Job drawing, mm, ordinate dimensions from the low corner. One solid piece. A direction names the side the tool comes from. Give positions to 0.01 mm unless a question says otherwise; leave off trailing zeros. Order: outer loops, then holes, each group sorted by start corner. A loop starts at its lowest first (then second) coordinate and runs counter-clockwise, first axis right, second up. Notation, with made-up numbers: (76, 37) -> (111, 37) arc R15 cw to (111, 44) -> close; hole circle Ø7 at (-4.75, 68). An arc over 180 degrees is marked (long way). Write item = value, one per line. Start each with the question number.
(1) Two-plate mould, pull along Y, no slides. Class the marked faces 3, 4 and 5: pulls with the +Y half, pulls with the -Y half, needs draft (parallel to the pull), parting line crosses it, or undercut.
(2) Saw through at B-B, the plane z = 4.2. List the corners of the cut face in (x, y), then the cut area to 3 significant figures.
(3) Probe line 1 along Y through (x, z) = (20, 0.2); line 2 along Y through (x, z) = (20, 1.6); line 3 along X through (y, z) = (29, 1.75) (1 decimal). List the from-to ranges inside material, lowest first. Write a range as from..to.
(4) Saw through at D-D, the plane x = 24. List the corners of the cut face in (y, z).
(5) Flat gauge pin, fed straight in: pin 1 (2 mm diameter, centred on y = 16.5, z = 4.5, fed in from -X). Where does the tip first touch, or does it go through?
(6) Saw through at A-A, the plane y = 20. List the corners of the cut face in (x, z).
(7) Saw through at C-C, the plane x = 20. List the corners of the cut face in (y, z).
(8) Which spindle directions (+Z, -Z, +X, -X, +Y, -Y) get a long thin tool onto all of the face, cutting with end or side? Do the marked faces 1 and 2. Say none if no direction does.
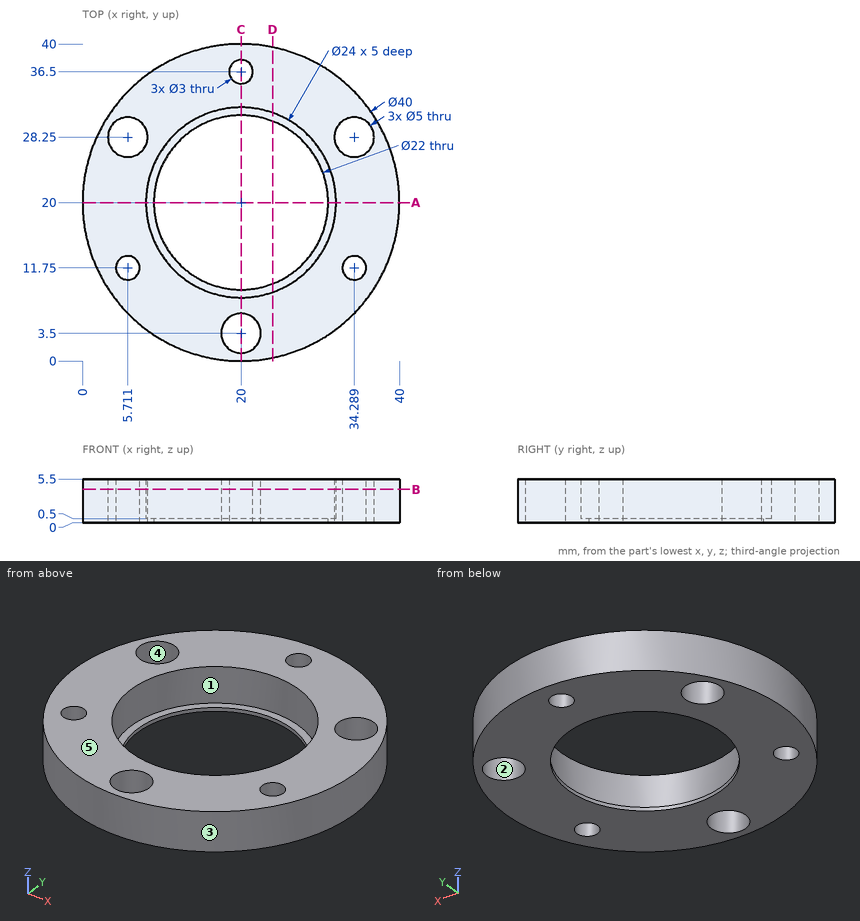
Results list:
q1.face_3 = parting line crosses it
q1.face_4 = undercut
q1.face_5 = needs draft
q2.outline = circle Ø40 at (20, 20); hole circle Ø5 at (5.71, 28.25); hole circle Ø3 at (5.71, 11.75); hole circle Ø24 at (20, 20); hole circle Ø5 at (20, 3.5); hole circle Ø3 at (20, 36.5); hole circle Ø5 at (34.29, 28.25); hole circle Ø3 at (34.29, 11.75)
q2.area = 724 mm^2
q3.line_1 = 0..1, 6..9, 31..35, 38..40
q3.line_2 = 0..1, 6..8, 32..35, 38..40
q3.line_3 = 2.1..3.3, 8.1..12.1, 27.9..31.9, 36.7..37.9
q4.outline = (0.4, 0) -> (9.75, 0) -> (9.75, 0.5) -> (8.69, 0.5) -> (8.69, 5.5) -> (0.4, 5.5) -> close; (30.25, 0) -> (39.6, 0) -> (39.6, 5.5) -> (31.31, 5.5) -> (31.31, 0.5) -> (30.25, 0.5) -> close
q5.pin_1 = 0.16
q6.outline = (0, 0) -> (9, 0) -> (9, 0.5) -> (8, 0.5) -> (8, 5.5) -> (0, 5.5) -> close; (31, 0) -> (40, 0) -> (40, 5.5) -> (32, 5.5) -> (32, 0.5) -> (31, 0.5) -> close
q7.outline = (0, 0) -> (1, 0) -> (1, 5.5) -> (0, 5.5) -> close; (6, 0) -> (9, 0) -> (9, 0.5) -> (8, 0.5) -> (8, 5.5) -> (6, 5.5) -> close; (31, 0) -> (35, 0) -> (35, 5.5) -> (32, 5.5) -> (32, 0.5) -> (31, 0.5) -> close; (38, 0) -> (40, 0) -> (40, 5.5) -> (38, 5.5) -> close
q8.face_1 = +Z
q8.face_2 = +Z, -Z
